Autodesk Inventor part; units mm, degrees
ref_plane "YZ Plane" through (0, 0, 0) normal (1, 0, 0) x (0, 1, 0)
ref_plane "XZ Plane" through (0, 0, 0) normal (0, 1, 0) x (-1, 0, 0)
ref_plane "XY Plane" through (0, 0, 0) normal (0, 0, 1) x (1, 0, 0)
sketch "Boceto1" plane through (0, 0, 0) normal (0, 0, 1) x (1, 0, 0)
  circle A0 centre (0, 0) radius 23.85
  circle A1 centre (0, 0) radius 26.85
  dimension "d0" = 47.7
  dimension "d1" = 3
extrude "Extrusión1" add sketch "Boceto1" along normal blind 9
sketch "Boceto2" plane through (0, 0, 0) normal (0, 0, -1) x (-1, 0, 0)
  circle A0 centre (0, 0) radius 37.5
  circle A1 centre (0, 0) radius 23.85
  dimension "d4" = 75
extrude "Extrusión2" add sketch "Boceto2" along normal blind 3
sketch "Boceto6" plane through (0, 0, 0) normal (0, 0, 1) x (1, 0, 0)
  circle A0 centre (0, 33) radius 1.8
  point P0 (0, 0)
  dimension "d19" = 3.6
  dimension "d20" = 33
extrude "Extrusión5" cut sketch "Boceto6" against normal blind 10
pattern_circular "Patrón circular1" count 4 over 360 about axis through (0, 0, -10) along (0, 0, 1) of "Extrusión5"
properties part number "AcoplecN°2"
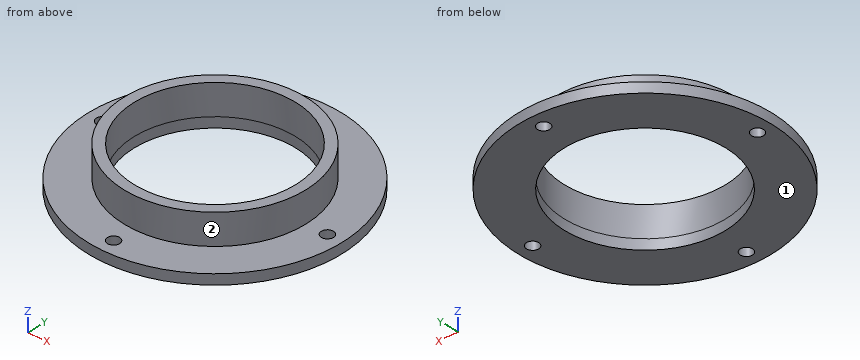
The listing builds one solid part. Answer for the finished solid, in the listing's coordinates (mm). Face numbers are marked on the shaded views. A direction names the side the tool comes from. Coordinates: 2 decimals unless noted, no trailing zeros. Loops run counter-clockwise (first coordinate to the right, second up) from the corner with the lowest first, then second, coordinate; pieces in that order, holes last. Notation, with made-up numbers: (31, -15) -> (71, -15) arc R20 cw to (71, 9) -> close; hole circle Ø5 at (88.5, 52.25). An arc over 180 degrees is marked (long way). Use one line per item in the form item = value. Start each with the question number.
Item 1: A tool of negligible diameter and unlimited length cuts with its end or side. For the marked faces 1 and 2, from which of +Z, -Z, +X, -X, +Y, -Y can it reach the whole face along a straight path? Write none if from no direction.
Item 2: Flat-ended cylindrical pins translate along their axes: pin 1 Ø6 at (x, y) = (0, -33) entering from +Z; pin 2 Ø5 at (x, z) = (1, 3.5) entering from -Y; pin 3 Ø1.5 at (x, z) = (-9.5, 5.5) entering from -Y; pin 4 Ø1.5 at (x, y) = (12, 17.5) entering from -Z. Find the tip coordinate at first contact, or state that the pin passes through.
Item 3: The part is cut by section C-C on y = 33. Determine the outline of the cut face in (x, z), then the cut area to 3 significant figures.
Item 4: The part is cut by section A-A on y = 0. Determine the outline of the cut face in (x, z), then the cut area to 3 significant figures.
Item 5: Consider L1, parallel to Y at x = 0, z = 8.5; L2, parallel to Z at x = -15, y = -25.5; L3, parallel to X at y = 18.5, z = 3. Determine where each line is inside the solid, lowest interval first. Write a range as [from, to].
Item 6: The part is cut by section D-D on z = -2. Determine the outline of the cut face in (x, y).
Answer key:
q1.face_1 = -Z, +X, -X, +Y, -Y
q1.face_2 = +Z
q2.pin_1 = 0
q2.pin_2 = -26.85
q2.pin_3 = -25.38
q2.pin_4 = through
q3.outline = (-17.81, -3) -> (-1.8, -3) -> (-1.8, 0) -> (-17.81, 0) -> close; (1.8, -3) -> (17.81, -3) -> (17.81, 0) -> (1.8, 0) -> close
q3.area = 96.1 mm2
q4.outline = (-37.5, -3) -> (-34.8, -3) -> (-34.8, 0) -> (-37.5, 0) -> close; (-31.2, -3) -> (-23.85, -3) -> (-23.85, 9) -> (-26.85, 9) -> (-26.85, 0) -> (-31.2, 0) -> close; (23.85, -3) -> (31.2, -3) -> (31.2, 0) -> (26.85, 0) -> (26.85, 9) -> (23.85, 9) -> close; (34.8, -3) -> (37.5, -3) -> (37.5, 0) -> (34.8, 0) -> close
q4.area = 114 mm2
q5.L1 = [-26.85, -23.85], [23.85, 26.85]
q5.L2 = [-3, 0]
q5.L3 = [-19.46, -15.05], [15.05, 19.46]
q6.outline = circle Ø75 at (0, 0); hole circle Ø3.6 at (-33, 0); hole circle Ø47.7 at (0, 0); hole circle Ø3.6 at (0, -33); hole circle Ø3.6 at (0, 33); hole circle Ø3.6 at (33, 0)
